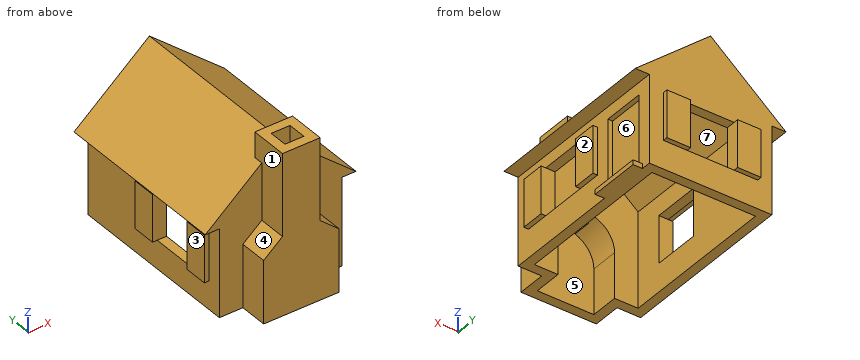
from build123d import *

# Parameters (mm, degrees)
F1_DEPTH       = 19
F2_W           = 10
F2_H           = 10
F3_DEPTH       = 19.001
F4_W           = 28
F4_H           = 20
F5_DEPTH       = 10
F6_W           = 10
F6_H           = 10
F7_DEPTH       = 16.001
F7_DEPTH_BACK  = 16.001
F8_W           = 5
F8_H           = 10
F9_DEPTH       = 1
F10_W          = 22
F10_H          = 34
F11_DEPTH      = 18.5754059012
F13_DEPTH      = 17
F13_DEPTH_BACK = 17
F14_W          = 8
F14_H          = 8
F15_DEPTH      = 34
F17_DEPTH      = 8
F18_W          = 4
F18_H          = 4
F19_DEPTH      = 34.001
F21_DEPTH      = 23
F22_W          = 9
F22_H          = 16
F23_DEPTH      = 1
F24_W          = 11
F24_H          = 1
F25_DEPTH      = 4


with BuildPart() as f1:
    # F0 (on Front) → F1 (new body, symmetric)
    with BuildSketch(Plane.XZ):
        Polygon((-13, 18.5744059012), (-13, 0), (13, 0), (13, 18.5744059012), (16, 18.5744059012), (0, 32), (-16, 18.5744059012), align=None)
    extrude(amount=F1_DEPTH, both=True)

    # F2 (on Front) → F3 (cut, through all)
    with BuildSketch(Plane.XZ):
        with Locations((0, 11)):
            Rectangle(F2_W, F2_H)
    extrude(amount=-F3_DEPTH, mode=Mode.SUBTRACT)

    # F4 (on face) → F5 (join, through all)
    with BuildSketch(Plane.XY.offset(6)):
        with Locations((0, -6)):
            Rectangle(F4_W, F4_H)
    extrude(amount=F5_DEPTH)

    # F6 (on Right) → F7 (cut, two sides)
    with BuildSketch(Plane.YZ) as f7_sk:
        with Locations((-6, 11)):
            Rectangle(F6_W, F6_H)
    extrude(amount=-F7_DEPTH, mode=Mode.SUBTRACT)
    extrude(f7_sk.sketch, amount=F7_DEPTH_BACK, mode=Mode.SUBTRACT)

    # F8 (on face) → F9 (join)
    with BuildSketch(Plane(origin=(0, 19, 0), x_dir=(-1, 0, 0), z_dir=(0, 1, 0))):
        with Locations((-7.5, 11)):
            Rectangle(F8_W, F8_H)
        with Locations((7.5, 11)):
            Rectangle(F8_W, F8_H)
    extrude(amount=F9_DEPTH)

    # F10 (on face) → F11 (cut, through all)
    with BuildSketch(Plane(origin=(0, 0, 18.5744059012), x_dir=(1, 0, 0), z_dir=(0, 0, -1))):
        Rectangle(F10_W, F10_H)
    extrude(amount=F11_DEPTH, mode=Mode.SUBTRACT)

    # F12 (on Front) → F13 (cut, two sides)
    with BuildSketch(Plane.XZ) as f13_sk:
        Polygon((-11, 20.1590894784), (-11, 18.5744059012), (11, 18.5744059012), (11, 20.1590894784), (0, 29.3891854213), align=None)
    extrude(amount=-F13_DEPTH, mode=Mode.SUBTRACT)
    extrude(f13_sk.sketch, amount=F13_DEPTH_BACK, mode=Mode.SUBTRACT)

    # F14 (on Top) → F15 (join)
    with BuildSketch(Plane.XY):
        with Locations((0, -21)):
            Rectangle(F14_W, F14_H)
    extrude(amount=F15_DEPTH)

    # F16 (on face) → F17 (join, through all)
    with BuildSketch(Plane.XZ.offset(25)):
        Polygon((8, 13.2872029506), (0, 20), (-8, 13.2872029506), (-8, 0), (8, 0), align=None)
    extrude(amount=-F17_DEPTH)

    # F18 (on face) → F19 (cut, through all)
    with BuildSketch(Plane.XY.offset(34)):
        with Locations((0, -21)):
            Rectangle(F18_W, F18_H)
    extrude(amount=-F19_DEPTH, mode=Mode.SUBTRACT)

    # F20 (on Front) → F21 (cut, through all)
    with BuildSketch(Plane.XZ):
        with BuildLine():
            ThreePointArc((6, 9.5567416853), (0, 15.5567416853), (-6, 9.5567416853))
            Line((-6, 9.5567416853), (-6, 0))
            Line((-6, 0), (6, 0))
            Line((6, 0), (6, 9.5567416853))
        make_face()
    extrude(amount=F21_DEPTH, mode=Mode.SUBTRACT)

    # F22 (on face) → F23 (cut)
    with BuildSketch(Plane.YZ.offset(13)):
        with Locations((11.5, 8)):
            Rectangle(F22_W, F22_H)
    extrude(amount=-F23_DEPTH, mode=Mode.SUBTRACT)

    # F24 (on face) → F25 (join)
    with BuildSketch(Plane(origin=(11, 0, 0), x_dir=(0, -1, 0), z_dir=(-1, 0, 0))):
        with Locations((-11.5, 0.5)):
            Rectangle(F24_W, F24_H)
    extrude(amount=-F25_DEPTH)


solid = f1.part
Check sheet for the modelled part. Datum: model origin and axes. Units: mm. Face numbers are marked on the shaded views. A direction names the side the tool comes from. Coordinates: 2 decimals unless noted, no trailing zeros. Write each loop counter-clockwise with the first axis right and the second up, starting at its lowest first coordinate (ties: lowest second). Pieces come first, ordered by that corner, then holes.
Item 1: Cross-section at D-D on x = -9. Record the boundary of the cut face in (y, z).
Numbers:
outline: (-19, 0) - (-17, 0) - (-17, 21.84) - (17, 21.84) - (17, 0) - (19, 0) - (19, 6) - (20, 6) - (20, 16) - (19, 16) - (19, 24.45) - (-19, 24.45) - close
Item 2: Cross-section at B-B on x = 3. Record the boundary of the cut face in (y, z), then the cut area to 3 significant figures.
Numbers:
outline: (-25, 0) - (-23, 0) - (-23, 14.75) - (-17, 14.75) - (-17, 26.87) - (17, 26.87) - (17, 16) - (19, 16) - (19, 29.48) - (-17, 29.48) - (-17, 34) - (-25, 34) - close; (17, 0) - (19, 0) - (19, 6) - (17, 6) - close
area: 311 mm2
Item 3: Access from +Z, -Z, +X, -X, +Y, -Y to the whole of each face (thin tool, end or side, straight path). Record for the marked faces 1, 2 and 3.
Numbers:
face 1: +Z, -X, -Y
face 2: -Z, +X, +Y, -Y
face 3: -Z, -X, +Y, -Y
Item 4: Cross-section at A-A on z = 3. Record the boundary of the cut face in (x, y).
Numbers:
outline: (-13, -19) - (-8, -19) - (-8, -25) - (8, -25) - (8, -19) - (13, -19) - (13, 7) - (12, 7) - (12, 16) - (13, 16) - (13, 19) - (-13, 19) - close; hole (-11, -17) - (-6, -17) - (-6, -23) - (6, -23) - (6, -17) - (11, -17) - (11, 17) - (-11, 17) - close
Item 5: Cross-section at C-C on y = 5. Record the boundary of the cut face in (x, z).
Numbers:
outline: (-16, 18.57) - (-13, 18.57) - (-13, 0) - (-11, 0) - (-11, 20.16) - (0, 29.39) - (11, 20.16) - (11, 0) - (13, 0) - (13, 18.57) - (16, 18.57) - (0, 32) - close
Item 6: Mould release check, pull along X, two halves, no side actions. Record for the marked faces 4, 5, 6 and 7: released by +X, released by -X, zero draft, split by the parting line, or undercut.
Numbers:
face 4: released by -X
face 5: undercut
face 6: released by +X
face 7: undercut
Item 7: Scan lines: probe 1 along Y at (x, z) = (-0.5, 28); probe 2 along Y at (x, z) = (6, 22); probe 3 along Y at (x, z) = (-3, 2). Record each from-to range of solid material in increasing order.
Numbers:
probe 1: y = -25 to -23, -19 to -17, 17 to 19
probe 2: y = -19 to -17, 17 to 19
probe 3: y = -25 to -23, 17 to 19
Item 8: Depth check by flat-ended pin: pin 1 Ø1.5 at (x, z) = (13, 13) entering from -Y; pin 2 Ø0.6 at (x, y) = (2, 17.5) entering from +Z; pin 3 Ø3 at (y, z) = (-18.5, 20) entering from +X. Enter the tip coordinate at first touch or a pass-through.
Numbers:
pin 1: stops at y = -19
pin 2: stops at z = 30.57
pin 3: stops at x = 16
